Model file for the job. Use its own axes, mm. A direction names the side the tool comes from. Coordinates: 2 decimals unless noted, no trailing zeros. Write each loop counter-clockwise with the first axis right and the second up, starting at its lowest first coordinate (ties: lowest second). Pieces come first, ordered by that corner, then holes. Notation, with made-up numbers: M 54,75 L 90,75 A19 ccw 90,89 Z; hole C 21.5,-3 d5. An arc over 180 degrees is marked long. Use CSV: the item, a comma, the result in double quotes. Start each with the question number.
from build123d import *

# Parameters (mm, degrees)
SKETCH_1_R                 = 2
EXTRUDE_1_DEPTH            = 12
SKETCH_2_R                 = 1.5
CUT_EXTRUDE_1_DEPTH        = 42.868842831
PATTERN_LINEAR_1_COUNT     = 2
PATTERN_LINEAR_1_PITCH     = 10
PATTERN_LINEAR_1_COL_COUNT = 2
PATTERN_LINEAR_1_COL_PITCH = 10
SKETCH_4_R                 = 7
EXTRUDE_2_DEPTH            = 25
SKETCH_7_R                 = 2
SKETCH_7_R_2               = 1
EXTRUDE_3_DEPTH            = 4
EXTRUDE_5_DEPTH            = 2
SKETCH_10_R                = 4.9
EXTRUDE_6_DEPTH            = 10
CUT_EXTRUDE_START          = -4
SKETCH_13_R                = 4.9
SKETCH_13_R_2              = 3
CUT_EXTRUDE_2_DEPTH        = 4


with BuildPart() as part:
    # 草图1 → 凸台-拉伸1 (new body)
    with BuildSketch(Plane.XY):
        with BuildLine():
            Line((0, 3), (37, 3))
            ThreePointArc((37, 3), (40, 0), (37, -3))
            Line((37, -3), (0, -3))
            ThreePointArc((0, -3), (-3, 0), (0, 3))
        make_face()
        Circle(SKETCH_1_R, mode=Mode.SUBTRACT)
        with Locations((37, 0)):
            Circle(SKETCH_1_R, mode=Mode.SUBTRACT)
    extrude(amount=EXTRUDE_1_DEPTH)

    # 草图2 → 切除-拉伸1 (cut, through all)
    with BuildSketch(Plane.XY.offset(12)):
        with Locations((18.5, 0)):
            Circle(SKETCH_2_R)
    cut_extrude_1 = extrude(amount=-CUT_EXTRUDE_1_DEPTH, mode=Mode.SUBTRACT)

    # 阵列(线性)1: 切除-拉伸1 ×2
    with Locations(*[(-i * PATTERN_LINEAR_1_PITCH, 0, 0) for i in range(1, PATTERN_LINEAR_1_COUNT)]):
        add(cut_extrude_1, mode=Mode.SUBTRACT)

    # 阵列(线性)1 col: 切除-拉伸1 ×2
    with Locations(*[(i * PATTERN_LINEAR_1_COL_PITCH, 0, 0) for i in range(1, PATTERN_LINEAR_1_COL_COUNT)]):
        add(cut_extrude_1, mode=Mode.SUBTRACT)

    # 草图4 → 凸台-拉伸2 (add)
    with BuildSketch(Plane(origin=(0, 3, 0), x_dir=(1, 0, 0), z_dir=(0, 1, 0))):
        with Locations(Location((18.5, -6, 0), (0, 0, 58.997280866))):
            Circle(SKETCH_4_R)
    extrude(amount=EXTRUDE_2_DEPTH)

    # 草图7 → 凸台-拉伸3 (add)
    with BuildSketch(Plane(origin=(0, 28, 0), x_dir=(1, 0, 0), z_dir=(0, 1, 0))):
        with Locations((11.5, -6)):
            Circle(SKETCH_7_R)
        with Locations((11.5, -6)):
            Circle(SKETCH_7_R_2, mode=Mode.SUBTRACT)
    extrude(amount=-EXTRUDE_3_DEPTH)

    # 草图9 → 凸台-拉伸5 (add, symmetric)
    with BuildSketch(Plane(origin=(0, 14, 0), x_dir=(-1, 0, 0), z_dir=(0, -1, 0))):
        with BuildLine():
            ThreePointArc((-11.785714286, -7.979486637), (-11.66092193, -7.492317377), (-11.571428571, -6.997445717))
            ThreePointArc((-11.571428571, -6.997445717), (-10.5, -6), (-11.571428571, -5.002554283))
            ThreePointArc((-11.571428571, -5.002554283), (-11.66092193, -4.507682623), (-11.785714286, -4.020513363))
            ThreePointArc((-11.785714286, -4.020513363), (-9.5, -6), (-11.785714286, -7.979486637))
        make_face()
    extrude(amount=EXTRUDE_5_DEPTH, both=True)

    # 草图10 → 凸台-拉伸6 (add)
    with BuildSketch(Plane(origin=(0, 28, 0), x_dir=(1, 0, 0), z_dir=(0, 1, 0))):
        with Locations(Location((18.5, -6, 0), (0, 0, 270))):
            Circle(SKETCH_10_R)
    extrude(amount=EXTRUDE_6_DEPTH)

    # 草图13 → 切除-拉伸2 (cut)
    with BuildSketch(Plane(origin=(0, 35.5, 0), x_dir=(1, 0, 0), z_dir=(0, 1, 0)).offset(CUT_EXTRUDE_START)):
        with Locations(Location((18.5, -6, 0), (0, 0, 270))):
            Circle(SKETCH_13_R)
        with Locations(Location((18.5, -6, 0), (0, 0, 270))):
            Circle(SKETCH_13_R_2, mode=Mode.SUBTRACT)
    extrude(amount=CUT_EXTRUDE_2_DEPTH, mode=Mode.SUBTRACT)


solid = part.part
1) Band-saw the part on D-D on x = 8. List the corners of the cut face in (y, z).
2) Band-saw the part on A-A on z = 6. State how many separate pieces and enclosed holes the cut face has, then the cut area to 3 significant figures.
3) Band-saw the part on B-B on x = 18.5. List the corners of the cut face in (y, z), then the cut area to 3 significant figures.
4) Drop flat-ended pins along their axis: P1, Ø5, axis at x = 21, y = 0, coming from the -Z side; P2, Ø3, axis at y = 7, z = 1.5, coming from the +X side; P3, Ø3.5, axis at x = 8.5, y = 0, coming from the +Z side; P4, Ø2.5, axis at x = 28.5, y = 0, coming from the -Z side. Give the stop position or say it passes through.
5) Band-saw the part on C-C on z = 2. List the corners of the cut face in (x, y), then the cut area to 3 significant figures.
6) Wall check: L1, parallel to Y at x = 8.5, z = 7.25; L2, parallel to Y at x = 18.5, z = 4; L3, parallel to Y at x = 34.5, z = 4. Give the ranges that are in metal, low to high. Write a range as [from, to].
7) Two-plate mould, pull along X, no slides. Class faces 1 (the face through (7, 0, 6)), 2 (the face through (10, 12, 6)), 3 (the face through (13.717, 36.732, 4.938)): pulls with the +X half, pulls with the -X half, needs draft (parallel to the pull), parting line crosses it, or undercut.
8) Tool access for faces 4 (the face through (18.6, 3, -0.6)), 5 (the face through (13.717, 29.726, 4.938)), 6 (the face through (35, 0, 6)): list every direction of +Z, -Z, +X, -X, +Y, -Y with a clear straight run to the whole face (end or side of a thin tool).
Findings below:
1,outline,"M -3,0 L -1.41,0 L -1.41,12 L -3,12 Z; M 1.41,0 L 3,0 L 3,12 L 1.41,12 Z"
2,separate pieces,"3"
2,enclosed holes,"5"
2,area,"645 mm2"
3,outline,"M -3,0 L -1.5,0 L -1.5,12 L -3,12 Z; M 1.5,0 L 3,0 L 3,-1 L 28,-1 L 28,1.1 L 31.5,1.1 L 31.5,3 L 35.5,3 L 35.5,1.1 L 38,1.1 L 38,10.9 L 35.5,10.9 L 35.5,9 L 31.5,9 L 31.5,10.9 L 28,10.9 L 28,13 L 3,13 L 3,12 L 1.5,12 Z"
3,area,"469 mm2"
4,P1,"stops at z = 0"
4,P2,"stops at x = 24.82"
4,P3,"stops at z = 12"
4,P4,"passes through"
5,outline,"M 0,-3 L 37,-3 A3 ccw 37,3 L 24.24,3 L 24.24,28 L 21.33,28 L 21.33,31.5 L 15.67,31.5 L 15.67,28 L 12.76,28 L 12.76,3 L 0,3 A3 ccw Z; M 15.67,35.5 L 21.33,35.5 L 21.33,38 L 15.67,38 Z; hole C 0,0 d4; hole C 8.5,0 d3; hole C 18.5,0 d3; hole C 28.5,0 d3; hole C 37,0 d4"
5,area,"525 mm2"
6,L1,"y = [-3, -1.5], [1.5, 3]"
6,L2,"y = [-3, -1.5], [1.5, 38]"
6,L3,"y = [-3, 3]"
7,face 1,"undercut"
7,face 2,"needs draft"
7,face 3,"parting line crosses it"
8,face 4,"-Z, +X, -X, -Y"
8,face 5,"+Y"
8,face 6,"+Z, -Z"
